from build123d import *

# Parameters (mm, degrees)
F1_DEPTH = 12.7
F2_R     = 2.65
F3_DEPTH = 51.816
F4_R     = 5.08
F5_W     = 6.35
F5_H     = 1.524
F6_DEPTH = 7.2898


with BuildPart() as f1:
    # F0 (on Top) → F1 (new body)
    with BuildSketch(Plane.XY):
        Polygon((16.51, 0), (0, 0), (0, -4.7625), (25.4, -4.7625), (31.75, -4.7625), (31.75, 15.1765), (0, 15.1765), (0, 10.414), (16.51, 10.414), align=None)
    extrude(amount=F1_DEPTH)

    # F2 (on face) → F3 (cut)
    with BuildSketch(Plane.XZ.offset(4.7625)):
        with Locations((5.588, 6.35)):
            Circle(F2_R)
    extrude(amount=-F3_DEPTH, mode=Mode.SUBTRACT)

    # F4
    f4_edges = [f1.edges().sort_by_distance(p)[0] for p in [
        (0, -2.38125, 12.7),
        (0, 12.79525, 12.7),
        (0, -2.38125, 0),
        (0, 12.79525, 0),
    ]]
    fillet(f4_edges, radius=F4_R)

    # F5 (on face) → F6 (cut)
    with BuildSketch(Plane.XZ.offset(4.7625)):
        Polygon((25.4, 7.112), (25.4, 14.78833), (23.368, 14.78833), (23.368, -2.12807), (25.4, -2.12807), (25.4, 5.588), align=None)
        with Locations((28.575, 6.35)):
            Rectangle(F5_W, F5_H)
    extrude(amount=-F6_DEPTH, mode=Mode.SUBTRACT)


solid = f1.part
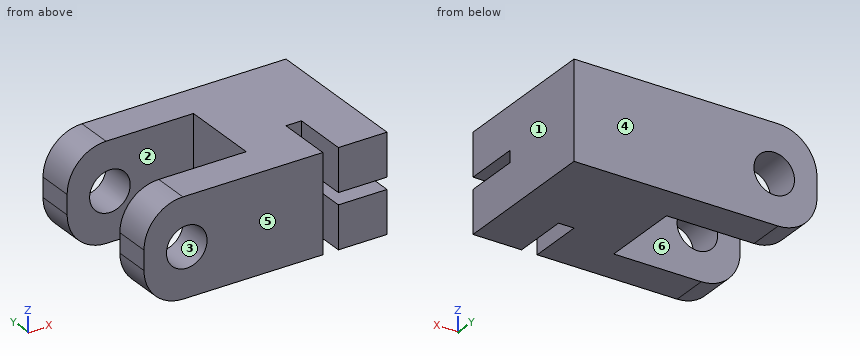
Input: part model. Units: mm. Frame: model coordinates. Face numbers are marked on the shaded views. A direction names the side the tool comes from. Give positions to 0.01 mm unless a question says otherwise; leave off trailing zeros. Order: outer loops, then holes, each group sorted by start corner. A loop starts at its lowest first (then second) coordinate and runs counter-clockwise, first axis right, second up.
Q1. Contact query for flat-ended pins moving along their axis: pin 1 Ø4.5 at (y, z) = (-2, 2.5) entering from -X; pin 2 Ø5 at (y, z) = (4.5, 9) entering from -X; pin 3 Ø2 at (y, z) = (-2, 3) entering from -X. Output: stop coordinate, or through.
Checked values:
pin 1: stops at x = 0.01
pin 2: stops at x = 16.51
pin 3: stops at x = 0.12
Q2. Section D-D on x = 4. Output: boundary loops of the cut face in (y, z), and give its area (3 significant figures).
Checked values:
outline: (-4.76, 0.12) - (0, 0.12) - (0, 4.23) - (-4.76, 4.23) - close; (-4.76, 8.47) - (0, 8.47) - (0, 12.58) - (-4.76, 12.58) - close; (10.41, 0.12) - (15.18, 0.12) - (15.18, 4.23) - (10.41, 4.23) - close; (10.41, 8.47) - (15.18, 8.47) - (15.18, 12.58) - (10.41, 12.58) - close
area: 78.3 mm2
Q3. Set-up query: the marked faces 1 and 2. Return all of +Z, -Z, +X, -X, +Y, -Y with unobstructed straight access to the full face (end or side cutting, diameter ignored); none if empty.
Checked values:
face 1: +Z, -Z, +X, +Y, -Y
face 2: +Z, -Z, -X
Q4. Section A-A on y = -3.5. Output: boundary loops of the cut face in (x, z), and give its area (3 significant figures).
Checked values:
outline: (0, 5.08) arc R5.08 ccw to (5.08, 0) - (23.37, 0) - (23.37, 12.7) - (5.08, 12.7) arc R5.08 ccw to (0, 7.62) - close; (25.4, 0) - (31.75, 0) - (31.75, 5.59) - (25.4, 5.59) - close; (25.4, 7.11) - (31.75, 7.11) - (31.75, 12.7) - (25.4, 12.7) - close; hole circle Ø5.3 at (5.59, 6.35)
area: 335 mm2
Q5. Ray query, probe 1 along Y at (x, z) = (14, 11.5); probe 2 along X at (y, z) = (-1.5, 7.75); probe 3 along X at (y, z) = (-0.25, 5.75). Return the intervals inside material, ascending.
Checked values:
probe 1: y = -4.76 to 0, 10.41 to 15.18
probe 2: x = 0 to 3.34, 7.84 to 23.37, 25.4 to 31.75
probe 3: x = 0 to 3.01, 8.17 to 23.37
Q6. Section C-C on y = 1. Output: boundary loops of the cut face in (x, z).
Checked values:
outline: (16.51, 0) - (23.37, 0) - (23.37, 12.7) - (16.51, 12.7) - close; (25.4, 0) - (31.75, 0) - (31.75, 5.59) - (25.4, 5.59) - close; (25.4, 7.11) - (31.75, 7.11) - (31.75, 12.7) - (25.4, 12.7) - close
Q7. Section B-B on z = 6.35. Output: boundary loops of the cut face in (x, y), and give its area (3 significant figures).
Checked values:
outline: (0, -4.76) - (2.94, -4.76) - (2.94, 0) - (0, 0) - close; (0, 10.41) - (2.94, 10.41) - (2.94, 15.18) - (0, 15.18) - close; (8.24, -4.76) - (23.37, -4.76) - (23.37, 2.53) - (31.75, 2.53) - (31.75, 15.18) - (8.24, 15.18) - (8.24, 10.41) - (16.51, 10.41) - (16.51, 0) - (8.24, 0) - close
area: 350 mm2
Q8. Draft query along Y for the marked faces 3, 4, 5 and 6. Return one class per face: +Y half, -Y half, draft (parallel to the pull), parting line (faces both ways), or undercut.
Checked values:
face 3: draft
face 4: +Y half
face 5: -Y half
face 6: undercut
